from build123d import *

# Parameters (mm, degrees)
SKETCH1_W           = 100
SKETCH1_H           = 50
BOSS_EXTRUDE1_DEPTH = 10
LPATTERN1_COUNT     = 2
LPATTERN1_PITCH     = 33.333333333


with BuildPart() as part:
    # Sketch1 → Boss-Extrude1 (new body)
    with BuildSketch(Plane.XY):
        Rectangle(SKETCH1_W, SKETCH1_H)
    extrude(amount=BOSS_EXTRUDE1_DEPTH)

    # Sketch2 → Ø20.0mm Dowel Slot1 (revolve, cut)
    with BuildSketch(Plane(origin=(-35, 0, 10), x_dir=(0, -1, 0), z_dir=(1, 0, 0))):
        Polygon((0, 0), (0, 16.00860619), (10, 10), (10, 0), align=None)
    f_20_0mm_dowel_slot1 = revolve(axis=Axis((-35, 0, 16.35), (0, 0, -1)), mode=Mode.SUBTRACT)

    # LPattern1: Ø20.0mm Dowel Slot1 ×2
    with Locations(*[(i * LPATTERN1_PITCH, 0, 0) for i in range(1, LPATTERN1_COUNT)]):
        add(f_20_0mm_dowel_slot1, mode=Mode.SUBTRACT)


solid = part.part
The model under review builds one solid part; all positions refer to its coordinate system, in mm. Round coordinates to 2 decimals unless told otherwise and drop trailing zeros. Write each loop counter-clockwise with the first axis right and the second up, starting at its lowest first coordinate (ties: lowest second). Pieces come first, ordered by that corner, then holes. Notation, with made-up numbers: (-31.5, 72.25) -> (-13.5, 72.25) arc R14 ccw to (-13.5, 86.25) -> close; hole circle Ø3 at (-33.75, 37.25). An arc over 180 degrees is marked (long way). Answer as a JSON object with one key per item and string values.
1. The part is to be moulded in two halves that separate along Y. For faces 1 (the face through (-1, 25, 5)), 2 (the face through (-50, 0, 5)), 3 (the face through (-25.24, 2.17, 5.07)), say which applies: pulls with the +Y half, pulls with the -Y half, needs draft (parallel to the pull), parting line crosses it, or undercut.
Results found:
{"face 1": "pulls with the +Y half", "face 2": "needs draft", "face 3": "undercut"}
2. We need section D-D on x = -9. State the section outline as (y, z) points, and give its area (3 significant figures).
Results found:
{"outline": "(-25, 0) -> (-6.8, 0) -> (-6.8, 10) -> (-25, 10) -> close; (6.8, 0) -> (25, 0) -> (25, 10) -> (6.8, 10) -> close", "area": "364 mm^2"}
3. We need section A-A on y = 0. State the section outline as (x, z) points.
Results found:
{"outline": "(-50, 0) -> (-45, 0) -> (-45, 10) -> (-50, 10) -> close; (-25, 0) -> (-11.67, 0) -> (-11.67, 10) -> (-25, 10) -> close; (8.33, 0) -> (50, 0) -> (50, 10) -> (8.33, 10) -> close"}
4. We need section C-C on z = 3.75. State the section outline as (x, y) points.
Results found:
{"outline": "(-50, -25) -> (50, -25) -> (50, 25) -> (-50, 25) -> close; hole circle Ø20 at (-35, 0); hole circle Ø20 at (-1.67, 0)"}
5. We need section B-B on x = -35. State the section outline as (y, z) points.
Results found:
{"outline": "(-25, 0) -> (-10, 0) -> (-10, 10) -> (-25, 10) -> close; (10, 0) -> (25, 0) -> (25, 10) -> (10, 10) -> close"}
6. To check wall thickness, follow line 1 along X through (y, z) = (0, 7.5); line 2 along X through (y, z) = (9, 1); line 3 along Y through (x, z) = (-35, 7.5). State the ranges of each line that lie inside material, in increasing order.
Results found:
{"line 1": "x = -50 to -45, -25 to -11.67, 8.33 to 50", "line 2": "x = -50 to -39.36, -30.64 to -6.03, 2.69 to 50", "line 3": "y = -25 to -10, 10 to 25"}
